from build123d import *

# Parameters (mm, degrees)
CUT_EXTRUDE_START   = -30
SKETCH_2_R          = 23.333333333
CUT_EXTRUDE_1_DEPTH = 30
CUT_EXTRUDE_2_DEPTH = 5


with BuildPart() as part:
    # Sketch 1 → Revolve 1 (revolve)
    with BuildSketch(Plane.XY, mode=Mode.PRIVATE) as revolve_1_sk:
        Polygon((0, 35), (14.208787172, 35), (15.933619666, 33.334348622), (16.923076923, 5), (17.5, 5), (17.5, 0), (8, 0), (6.9175, 1.0825), (6.9175, 23.5), (0, 23.5), align=None)
    revolve(revolve_1_sk.sketch.rotate(Axis((0, 0, 0), (0, 1, 0)), 270), axis=Axis((0, 0, 0), (0, 1, 0)))

    # Sketch 2 → Cut-Extrude 1 (cut)
    with BuildSketch(Plane(origin=(0, 35, 0), x_dir=(1, 0, 0), z_dir=(0, 1, 0)).offset(CUT_EXTRUDE_START)):
        Circle(SKETCH_2_R)
        with BuildLine():
            Line((-17.420454134, -1.666666667), (-14.90711985, -1.666666667))
            ThreePointArc((-14.90711985, -1.666666667), (-14.488887394, -3.882285677), (-13.743277821, -6.010184252))
            Line((-13.743277821, -6.010184252), (-15.919889159, -7.266851394))
            ThreePointArc((-15.919889159, -7.266851394), (-15.155444566, -8.75), (-14.253222492, -10.15360274))
            Line((-14.253222492, -10.15360274), (-12.076611154, -8.896935598))
            ThreePointArc((-12.076611154, -8.896935598), (-10.606601718, -10.606601718), (-8.896935598, -12.076611154))
            Line((-8.896935598, -12.076611154), (-10.15360274, -14.253222492))
            ThreePointArc((-10.15360274, -14.253222492), (-8.75, -15.155444566), (-7.266851394, -15.919889159))
            Line((-7.266851394, -15.919889159), (-6.010184252, -13.743277821))
            ThreePointArc((-6.010184252, -13.743277821), (-3.882285677, -14.488887394), (-1.666666667, -14.90711985))
            Line((-1.666666667, -14.90711985), (-1.666666667, -17.420454134))
            ThreePointArc((-1.666666667, -17.420454134), (0, -17.5), (1.666666667, -17.420454134))
            Line((1.666666667, -17.420454134), (1.666666667, -14.90711985))
            ThreePointArc((1.666666667, -14.90711985), (3.882285677, -14.488887394), (6.010184252, -13.743277821))
            Line((6.010184252, -13.743277821), (7.266851394, -15.919889159))
            ThreePointArc((7.266851394, -15.919889159), (8.75, -15.155444566), (10.15360274, -14.253222492))
            Line((10.15360274, -14.253222492), (8.896935598, -12.076611154))
            ThreePointArc((8.896935598, -12.076611154), (10.606601718, -10.606601718), (12.076611154, -8.896935598))
            Line((12.076611154, -8.896935598), (14.253222492, -10.15360274))
            ThreePointArc((14.253222492, -10.15360274), (15.155444566, -8.75), (15.919889159, -7.266851394))
            Line((15.919889159, -7.266851394), (13.743277821, -6.010184252))
            ThreePointArc((13.743277821, -6.010184252), (14.488887394, -3.882285677), (14.90711985, -1.666666667))
            Line((14.90711985, -1.666666667), (17.420454134, -1.666666667))
            ThreePointArc((17.420454134, -1.666666667), (17.5, 0), (17.420454134, 1.666666667))
            Line((17.420454134, 1.666666667), (14.90711985, 1.666666667))
            ThreePointArc((14.90711985, 1.666666667), (14.488887394, 3.882285677), (13.743277821, 6.010184252))
            Line((13.743277821, 6.010184252), (15.919889159, 7.266851394))
            ThreePointArc((15.919889159, 7.266851394), (15.155444566, 8.75), (14.253222492, 10.15360274))
            Line((14.253222492, 10.15360274), (12.076611154, 8.896935598))
            ThreePointArc((12.076611154, 8.896935598), (10.606601718, 10.606601718), (8.896935598, 12.076611154))
            Line((8.896935598, 12.076611154), (10.15360274, 14.253222492))
            ThreePointArc((10.15360274, 14.253222492), (8.75, 15.155444566), (7.266851394, 15.919889159))
            Line((7.266851394, 15.919889159), (6.010184252, 13.743277821))
            ThreePointArc((6.010184252, 13.743277821), (3.882285677, 14.488887394), (1.666666667, 14.90711985))
            Line((1.666666667, 14.90711985), (1.666666667, 17.420454134))
            ThreePointArc((1.666666667, 17.420454134), (0, 17.5), (-1.666666667, 17.420454134))
            Line((-1.666666667, 17.420454134), (-1.666666667, 14.90711985))
            ThreePointArc((-1.666666667, 14.90711985), (-3.882285677, 14.488887394), (-6.010184252, 13.743277821))
            Line((-6.010184252, 13.743277821), (-7.266851394, 15.919889159))
            ThreePointArc((-7.266851394, 15.919889159), (-8.75, 15.155444566), (-10.15360274, 14.253222492))
            Line((-10.15360274, 14.253222492), (-8.896935598, 12.076611154))
            ThreePointArc((-8.896935598, 12.076611154), (-10.606601718, 10.606601718), (-12.076611154, 8.896935598))
            Line((-12.076611154, 8.896935598), (-14.253222492, 10.15360274))
            ThreePointArc((-14.253222492, 10.15360274), (-15.155444566, 8.75), (-15.919889159, 7.266851394))
            Line((-15.919889159, 7.266851394), (-13.743277821, 6.010184252))
            ThreePointArc((-13.743277821, 6.010184252), (-14.488887394, 3.882285677), (-14.90711985, 1.666666667))
            Line((-14.90711985, 1.666666667), (-17.420454134, 1.666666667))
            ThreePointArc((-17.420454134, 1.666666667), (-17.5, 0), (-17.420454134, -1.666666667))
        make_face(mode=Mode.SUBTRACT)
    extrude(amount=CUT_EXTRUDE_1_DEPTH, mode=Mode.SUBTRACT)

    # Sketch 3 → Cut-Extrude 2 (cut)
    with BuildSketch(Plane(origin=(0, 23.5, 0), x_dir=(1, 0, 0), z_dir=(0, 1, 0))):
        with BuildLine():
            Line((1.538461538, -2.757795363), (1.538461538, 2.757795363))
            ThreePointArc((1.538461538, 2.757795363), (0, 3.157894737), (-1.538461538, 2.757795363))
            Line((-1.538461538, 2.757795363), (-1.538461538, -2.757795363))
            ThreePointArc((-1.538461538, -2.757795363), (0, -3.157894737), (1.538461538, -2.757795363))
        make_face()
    extrude(amount=CUT_EXTRUDE_2_DEPTH, mode=Mode.SUBTRACT)


solid = part.part
The listing builds one solid part. Answer for the finished solid, in the listing's coordinates (mm). A direction names the side the tool comes from. Round coordinates to 2 decimals unless told otherwise and drop trailing zeros. Write each loop counter-clockwise with the first axis right and the second up, starting at its lowest first coordinate (ties: lowest second). Pieces come first, ordered by that corner, then holes. Notation, with made-up numbers: (30, 81) - (69, 81) arc R32 cw to (69, 112) - close; hole circle Ø4 at (9.5, 60.25). An arc over 180 degrees is marked (long way). Use a Markdown table: item, result. Add a question column.
1. The part is cut by section A-A (z = 0). Write down the section's boundary in (x, y).
2. For a pull along X with two mould halves and no side action, classify faces 4 (the face through (-12.74, 16.16, 9.28)), 5 (the face through (14.38, 19.41, -6.38)), 6 (the face through (-16.435, 18.969, -0.024)), 7 (the face through (16, 16, -1.667)) as +X half, -X half, draft (parallel to the pull), parting line (faces both ways), or undercut.
3. Consider line 1 (Z direction, x = -9, y = 32); line 2 (Y direction, x = 15, z = 3); line 3 (Y direction, x = 3, z = 0.5). Determine where each line is inside the solid, lowest interval first.
4. A tool of negligible diameter and unlimited length cuts with its end or side. For faces 1 (the face through (-12.72, 19.41, -9.27)), 2 (the face through (10.629, 19.413, -10.584)), 3 (the face through (-0.022, 25.965, 3.158)), from which of +Z, -Z, +X, -X, +Y, -Y can it reach the whole face along a straight path? Write none if from no direction.
5. The part is cut by section B-B (x = 0). Write down the section's boundary in (y, z), and give its area (3 significant figures).
6. Flat-ended cylindrical pins translate along their axes: P1, Ø5, axis at y = 5.5, z = 13.5, coming from the -X side; P2, Ø4, axis at x = -1.5, y = 15, coming from the -Z side; P3, Ø2, axis at y = 16.5, z = -15.5, coming from the +X side; P4, Ø8, axis at x = 4.5, z = -10, coming from the -Y side. Find the tip coordinate at first contact, or state that the pin passes through.
Reported:
| question | item | result |
|---|---|---|
| 1 | outline | (-17.5, 0) - (-8, 0) - (-6.92, 1.08) - (-6.92, 23.5) - (-1.54, 23.5) - (-1.54, 28.5) - (1.54, 28.5) - (1.54, 23.5) - (6.92, 23.5) - (6.92, 1.08) - (8, 0) - (17.5, 0) - (17.5, 5) - (16.92, 5) - (15.93, 33.33) - (14.21, 35) - (-14.21, 35) - (-15.93, 33.33) - (-16.92, 5) - (-17.5, 5) - close |
| 2 | face 4 | undercut |
| 2 | face 5 | +X half |
| 2 | face 6 | -X half |
| 2 | face 7 | draft |
| 3 | line 1 | -13.2 to -12.26, -12 to 12, 12.26 to 13.2 |
| 3 | line 2 | 0 to 5 |
| 3 | line 3 | 23.5 to 35 |
| 4 | face 1 | -Z, +Y |
| 4 | face 2 | +Y |
| 4 | face 3 | -Y |
| 5 | outline | (0, -17.5) - (5, -17.5) - (5, -16.92) - (33.33, -15.93) - (35, -14.21) - (35, 14.21) - (33.33, 15.93) - (5, 16.92) - (5, 17.5) - (0, 17.5) - (0, 8) - (1.08, 6.92) - (23.5, 6.92) - (23.5, 3.16) - (28.5, 3.16) - (28.5, -3.16) - (23.5, -3.16) - (23.5, -6.92) - (1.08, -6.92) - (0, -8) - close |
| 5 | area | 798 mm^2 |
| 6 | P1 | x = -13.57 |
| 6 | P2 | z = -16.63 |
| 6 | P3 | x = 7.92 |
| 6 | P4 | y = 0 |
